Work out the finished part from the listing and answer in its coordinate system (mm). Give positions to 0.01 mm unless a question says otherwise; leave off trailing zeros. Write each loop counter-clockwise with the first axis right and the second up, starting at its lowest first coordinate (ties: lowest second). Pieces come first, ordered by that corner, then holes. Notation, with made-up numbers: (79, 16.5) - (129, 16.5) arc R32 cw to (129, 55.5) - close; hole circle Ø5 at (72.5, 83). An arc over 180 degrees is marked (long way). Write item = value, one per line.
from build123d import *

# Parameters (mm, degrees)
SKETCH_1_R          = 1.65
EXTRUDE_1_DEPTH     = 3
CUT_EXTRUDE_1_DEPTH = 3
FILLET_1_R          = 2
SKETCH_3_R          = 1
CUT_EXTRUDE_2_DEPTH = 3
CUT_EXTRUDE_3_DEPTH = 3


with BuildPart() as part:
    # 草图1 → 凸台-拉伸1 (new body)
    with BuildSketch(Plane(origin=(0, 0, 0), x_dir=(1, 0, 0), z_dir=(0, 1, 0))):
        with BuildLine():
            Line((-30, 20.5), (-15, 20.5))
            Line((-15, 20.5), (-15, 17.5))
            Line((-15, 17.5), (15, 17.5))
            Line((15, 17.5), (15, 20.5))
            Line((15, 20.5), (30, 20.5))
            Line((30, 20.5), (30, 17.5))
            Line((30, 17.5), (43, 17.5))
            ThreePointArc((43, 17.5), (44.414213562, 16.914213562), (45, 15.5))
            Line((45, 15.5), (45, -5.5))
            ThreePointArc((45, -5.5), (45.292893219, -6.207106781), (46, -6.5))
            Line((46, -6.5), (49.9, -6.5))
            ThreePointArc((49.9, -6.5), (50.607106781, -6.792893219), (50.9, -7.5))
            Line((50.9, -7.5), (50.9, -9.5))
            ThreePointArc((50.9, -9.5), (51.192893219, -10.207106781), (51.9, -10.5))
            Line((51.9, -10.5), (53.1, -10.5))
            ThreePointArc((53.1, -10.5), (53.807106781, -10.207106781), (54.1, -9.5))
            Line((54.1, -9.5), (54.1, -7.5))
            ThreePointArc((54.1, -7.5), (54.392893219, -6.792893219), (55.1, -6.5))
            Line((55.1, -6.5), (58.1, -6.5))
            ThreePointArc((58.1, -6.5), (58.807106781, -6.792893219), (59.1, -7.5))
            Line((59.1, -7.5), (59.1, -16.5))
            ThreePointArc((59.1, -16.5), (58.807106781, -17.207106781), (58.1, -17.5))
            Line((58.1, -17.5), (30, -17.5))
            Line((30, -17.5), (30, -20.5))
            Line((30, -20.5), (15, -20.5))
            Line((15, -20.5), (15, -17.5))
            Line((15, -17.5), (-15, -17.5))
            Line((-15, -17.5), (-15, -20.5))
            Line((-15, -20.5), (-30, -20.5))
            Line((-30, -20.5), (-30, -17.5))
            Line((-30, -17.5), (-34, -17.5))
            ThreePointArc((-34, -17.5), (-35.414213562, -16.914213562), (-36, -15.5))
            Line((-36, -15.5), (-36, 15.5))
            ThreePointArc((-36, 15.5), (-35.414213562, 16.914213562), (-34, 17.5))
            Line((-34, 17.5), (-30, 17.5))
            Line((-30, 17.5), (-30, 20.5))
        make_face()
        with Locations(Location((-9, 6, 0), (0, 0, 270))):
            Circle(SKETCH_1_R, mode=Mode.SUBTRACT)
        with Locations(Location((-9, -6, 0), (0, 0, 270))):
            Circle(SKETCH_1_R, mode=Mode.SUBTRACT)
    extrude(amount=EXTRUDE_1_DEPTH)

    # 草图2 → 切除-拉伸1 (cut)
    with BuildSketch(Plane(origin=(0, 3, 0), x_dir=(1, 0, 0), z_dir=(0, 1, 0))):
        with BuildLine():
            Line((37, -4), (45, -4))
            Line((45, -4), (45, 4))
            Line((45, 4), (37, 4))
            ThreePointArc((37, 4), (35.585786438, 3.414213562), (35, 2))
            Line((35, 2), (35, -2))
            ThreePointArc((35, -2), (35.585786438, -3.414213562), (37, -4))
        make_face()
    extrude(amount=-CUT_EXTRUDE_1_DEPTH, mode=Mode.SUBTRACT)

    # 圆角1
    fillet_1_edges = [part.edges().sort_by_distance(p)[0] for p in [
        (45, 1.5, 4),
        (45, 1.5, -4),
    ]]
    fillet(fillet_1_edges, radius=FILLET_1_R)

    # 草图3 → 切除-拉伸2 (cut)
    with BuildSketch(Plane(origin=(0, 3, 0), x_dir=(1, 0, 0), z_dir=(0, 1, 0))):
        with Locations((-31, 17.5)):
            Circle(SKETCH_3_R)
        with Locations((-14, 17.5)):
            Circle(SKETCH_3_R)
        with Locations((14, 17.5)):
            Circle(SKETCH_3_R)
        with Locations((31, 17.5)):
            Circle(SKETCH_3_R)
        with Locations((-31, -17.5)):
            Circle(SKETCH_3_R)
        with Locations((-14, -17.5)):
            Circle(SKETCH_3_R)
        with Locations((14, -17.5)):
            Circle(SKETCH_3_R)
        with Locations((31, -17.5)):
            Circle(SKETCH_3_R)
    extrude(amount=-CUT_EXTRUDE_2_DEPTH, mode=Mode.SUBTRACT)

    # 草图4 → 切除-拉伸3 (cut)
    with BuildSketch(Plane(origin=(0, 3, 0), x_dir=(1, 0, 0), z_dir=(0, 1, 0))):
        with BuildLine():
            Line((-15.360471904, 0.5), (-21.133974596, 10.5))
            ThreePointArc((-21.133974596, 10.5), (-21.133974596, 11.5), (-20.267949192, 12))
            Line((-20.267949192, 12), (-17.577350269, 12))
            ThreePointArc((-17.577350269, 12), (-17.077350269, 11.866025404), (-16.711324865, 11.5))
            Line((-16.711324865, 11.5), (-10.360471904, 0.5))
            ThreePointArc((-10.360471904, 0.5), (-10.226497308, 0), (-10.360471904, -0.5))
            Line((-10.360471904, -0.5), (-16.711324865, -11.5))
            ThreePointArc((-16.711324865, -11.5), (-17.077350269, -11.866025404), (-17.577350269, -12))
            Line((-17.577350269, -12), (-20.267949192, -12))
            ThreePointArc((-20.267949192, -12), (-21.133974596, -11.5), (-21.133974596, -10.5))
            Line((-21.133974596, -10.5), (-15.360471904, -0.5))
            ThreePointArc((-15.360471904, -0.5), (-15.226497308, 0), (-15.360471904, 0.5))
        make_face()
        with BuildLine():
            Line((-31.267949192, 12), (-28.577350269, 12))
            ThreePointArc((-28.577350269, 12), (-28.077350269, 11.866025404), (-27.711324865, 11.5))
            Line((-27.711324865, 11.5), (-21.360471904, 0.5))
            ThreePointArc((-21.360471904, 0.5), (-21.226497308, 0), (-21.360471904, -0.5))
            Line((-21.360471904, -0.5), (-27.711324865, -11.5))
            ThreePointArc((-27.711324865, -11.5), (-28.077350269, -11.866025404), (-28.577350269, -12))
            Line((-28.577350269, -12), (-31.267949192, -12))
            ThreePointArc((-31.267949192, -12), (-32.133974596, -11.5), (-32.133974596, -10.5))
            Line((-32.133974596, -10.5), (-26.360471904, -0.5))
            ThreePointArc((-26.360471904, -0.5), (-26.226497308, 0), (-26.360471904, 0.5))
            Line((-26.360471904, 0.5), (-32.133974596, 10.5))
            ThreePointArc((-32.133974596, 10.5), (-32.133974596, 11.5), (-31.267949192, 12))
        make_face()
        with BuildLine():
            Line((10.639528096, 0.5), (4.866025404, 10.5))
            ThreePointArc((4.866025404, 10.5), (4.866025404, 11.5), (5.732050808, 12))
            Line((5.732050808, 12), (8.422649731, 12))
            ThreePointArc((8.422649731, 12), (8.922649731, 11.866025404), (9.288675135, 11.5))
            Line((9.288675135, 11.5), (15.639528096, 0.5))
            ThreePointArc((15.639528096, 0.5), (15.773502692, 0), (15.639528096, -0.5))
            Line((15.639528096, -0.5), (9.288675135, -11.5))
            ThreePointArc((9.288675135, -11.5), (8.922649731, -11.866025404), (8.422649731, -12))
            Line((8.422649731, -12), (5.732050808, -12))
            ThreePointArc((5.732050808, -12), (4.866025404, -11.5), (4.866025404, -10.5))
            Line((4.866025404, -10.5), (10.639528096, -0.5))
            ThreePointArc((10.639528096, -0.5), (10.773502692, 0), (10.639528096, 0.5))
        make_face()
        with BuildLine():
            Line((-0.360471904, 0.5), (-6.133974596, 10.5))
            ThreePointArc((-6.133974596, 10.5), (-6.133974596, 11.5), (-5.267949192, 12))
            Line((-5.267949192, 12), (-2.577350269, 12))
            ThreePointArc((-2.577350269, 12), (-2.077350269, 11.866025404), (-1.711324865, 11.5))
            Line((-1.711324865, 11.5), (4.639528096, 0.5))
            ThreePointArc((4.639528096, 0.5), (4.773502692, 0), (4.639528096, -0.5))
            Line((4.639528096, -0.5), (-1.711324865, -11.5))
            ThreePointArc((-1.711324865, -11.5), (-2.077350269, -11.866025404), (-2.577350269, -12))
            Line((-2.577350269, -12), (-5.267949192, -12))
            ThreePointArc((-5.267949192, -12), (-6.133974596, -11.5), (-6.133974596, -10.5))
            Line((-6.133974596, -10.5), (-0.360471904, -0.5))
            ThreePointArc((-0.360471904, -0.5), (-0.226497308, 0), (-0.360471904, 0.5))
        make_face()
        with BuildLine():
            Line((23.639528096, 0.5), (17.866025404, 10.5))
            ThreePointArc((17.866025404, 10.5), (17.866025404, 11.5), (18.732050808, 12))
            Line((18.732050808, 12), (21.422649731, 12))
            ThreePointArc((21.422649731, 12), (21.922649731, 11.866025404), (22.288675135, 11.5))
            Line((22.288675135, 11.5), (28.639528096, 0.5))
            ThreePointArc((28.639528096, 0.5), (28.773502692, 0), (28.639528096, -0.5))
            Line((28.639528096, -0.5), (22.288675135, -11.5))
            ThreePointArc((22.288675135, -11.5), (21.922649731, -11.866025404), (21.422649731, -12))
            Line((21.422649731, -12), (18.732050808, -12))
            ThreePointArc((18.732050808, -12), (17.866025404, -11.5), (17.866025404, -10.5))
            Line((17.866025404, -10.5), (23.639528096, -0.5))
            ThreePointArc((23.639528096, -0.5), (23.773502692, 0), (23.639528096, 0.5))
        make_face()
        with BuildLine():
            Line((30.866025404, 13.5), (40.639528096, 13.5))
            ThreePointArc((40.639528096, 13.5), (41.346634877, 13.207106781), (41.639528096, 12.5))
            Line((41.639528096, 12.5), (41.639528096, 8.5))
            ThreePointArc((41.639528096, 8.5), (41.346634877, 7.792893219), (40.639528096, 7.5))
            Line((40.639528096, 7.5), (33.175426481, 7.5))
            ThreePointArc((33.175426481, 7.5), (32.675426481, 7.633974596), (32.309401077, 8))
            Line((32.309401077, 8), (30, 12))
            ThreePointArc((30, 12), (30, 13), (30.866025404, 13.5))
        make_face()
        with BuildLine():
            Line((32.886751346, -8), (39.339745962, -8))
            ThreePointArc((39.339745962, -8), (39.598565007, -8.034074174), (39.839745962, -8.133974596))
            Line((39.839745962, -8.133974596), (45.901923789, -11.633974596))
            ThreePointArc((45.901923789, -11.633974596), (46.367849615, -12.758819045), (45.401923789, -13.5))
            Line((45.401923789, -13.5), (30.866025404, -13.5))
            ThreePointArc((30.866025404, -13.5), (30, -13), (30, -12))
            Line((30, -12), (32.020725942, -8.5))
            ThreePointArc((32.020725942, -8.5), (32.386751346, -8.133974596), (32.886751346, -8))
        make_face()
    extrude(amount=-CUT_EXTRUDE_3_DEPTH, mode=Mode.SUBTRACT)


solid = part.part
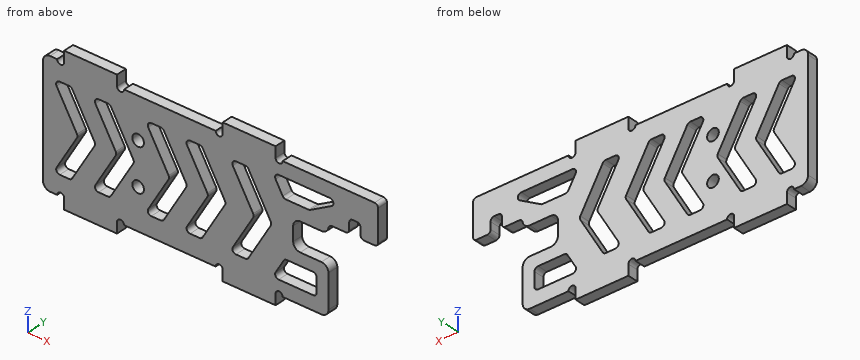
1. Find section A-A, the plane x = -9. Give the vertices of the cut face in (y, z).
Solution:
outline = (0, -17.5) - (3, -17.5) - (3, -7.65) - (0, -7.65) - close; (0, -4.35) - (3, -4.35) - (3, 4.35) - (0, 4.35) - close; (0, 7.65) - (3, 7.65) - (3, 17.5) - (0, 17.5) - close
2. Find section C-C, the plane y = 0.5. Give the number of separate pieces and of enclosed holes in the cut face, then the cut area to 3 significant figures.
Solution:
separate_pieces = 1
enclosed_holes = 9
area = 2,320 mm^2
3. Straight lines are drawn through the part: line 1 (Z direction, x = 39.5, y = 2.55); line 2 (Z direction, x = 33, y = 0.7); line 3 (X direction, y = 1.1, z = 2). For each, find the intervals that lie inside material, in ascending order.
Solution:
line_1 = -17.5 to -13.5, -7.5 to -4, 4 to 8.01, 13.5 to 17.5
line_2 = -17.5 to -13.5, -7.52 to 8, 13.5 to 17.5
line_3 = -36 to -27.23, -22.23 to -16.23, -11.23 to -1.23, 3.77 to 9.77, 14.77 to 22.77, 27.77 to 35
4. Find section B-B, the plane x = 14. Give the vertices of the cut face in (y, z), then the cut area to 3 significant figures.
Solution:
outline = (0, -16.5) - (3, -16.5) - (3, -3.34) - (0, -3.34) - close; (0, 3.34) - (3, 3.34) - (3, 16.5) - (0, 16.5) - close
area = 79.0 mm^2
5. Given pin 1 (0.9 mm diameter, centred on y = 1, z = 19.5, fed in from -X); pin 2 (1.5 mm diameter, centred on x = 45, y = 2, fed in from -Z); pin 3 (1.3 mm diameter, centred on x = 6.5, y = 2, fed in from +Z), each flat-ended and moving along its own axis, determine where each tip first touches the part or whether it passes through.
Solution:
pin_1 = -30
pin_2 = -17.06
pin_3 = 17.5
6. Find section D-D, the plane x = 48. Give the vertices of the cut face in (y, z).
Solution:
outline = (0, 6.5) - (3, 6.5) - (3, 17.5) - (0, 17.5) - close
